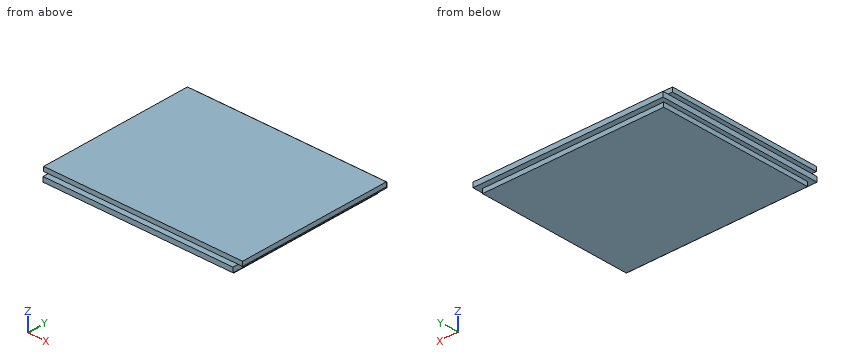
```python
from build123d import *

# Parameters (mm, degrees)
F0_W     = 114.3
F0_H     = 88.9
F1_DEPTH = 2.54
F2_W     = 109.22
F2_H     = 3.175
F2_H_2   = 88.9
F3_DEPTH = 2.794
F4_W     = 104.14
F4_H     = 88.9
F5_DEPTH = 2.54


with BuildPart() as f1:
    # F0 (on Top) → F1 (new body)
    with BuildSketch(Plane.XY):
        Rectangle(F0_W, F0_H)
    extrude(amount=-F1_DEPTH)

    # F2 (on face) → F3 (join)
    with BuildSketch(Plane(origin=(0, 0, -2.54), x_dir=(1, 0, 0), z_dir=(0, 0, -1))):
        with Locations((0, 46.0375)):
            Rectangle(F2_W, F2_H)
        Rectangle(F2_W, F2_H_2)
        with Locations((0, -46.0375)):
            Rectangle(F2_W, F2_H)
    extrude(amount=F3_DEPTH)

    # F4 (on face) → F5 (join)
    with BuildSketch(Plane(origin=(0, 0, -5.334), x_dir=(1, 0, 0), z_dir=(0, 0, -1))):
        Rectangle(F4_W, F4_H)
    extrude(amount=F5_DEPTH)


solid = f1.part
```
Model file for the job. Use its own axes, mm. Give positions to 0.01 mm unless a question says otherwise; leave off trailing zeros. Loops run counter-clockwise (first coordinate to the right, second up) from the corner with the lowest first, then second, coordinate; pieces in that order, holes last. Notation, with made-up numbers: (33.25, 88.5) -> (39.25, 88.5) arc R32 cw to (39.25, 116.5) -> close; hole circle Ø2 at (62.5, 3.5). An arc over 180 degrees is marked (long way). Write each question's results on one line, items separated by ' | '.
(1) Flat gauge pins, fed straight in: pin 1 Ø1.4 at (y, z) = (5.5, -4.5) entering from -X; pin 2 Ø0.8 at (y, z) = (1.5, -3.5) entering from +X; pin 3 Ø3 at (x, y) = (55.5, -0.5) entering from -Z. Where does each tip first touch, or does it go through?
Geometry results:
pin 1: stops at x = -54.61 | pin 2: stops at x = 54.61 | pin 3: stops at z = -5.33
(2) Cut at C-C on z = -1.25. List the corners of the cut face in (x, y), and give its area (3 significant figures).
Geometry results:
outline: (-57.15, -44.45) -> (57.15, -44.45) -> (57.15, 44.45) -> (-57.15, 44.45) -> close | area: 10,200 mm²
(3) Cut at B-B on x = -19. List the corners of the cut face in (y, z) (3 decimals), and give its area (3 significant figures).
Geometry results:
outline: (-47.625, -5.334) -> (-44.45, -5.334) -> (-44.45, -7.874) -> (44.45, -7.874) -> (44.45, -5.334) -> (47.625, -5.334) -> (47.625, -2.54) -> (44.45, -2.54) -> (44.45, 0) -> (-44.45, 0) -> (-44.45, -2.54) -> (-47.625, -2.54) -> close | area: 718 mm²
(4) Cut at A-A on y = -22. List the corners of the cut face in (x, z), and give its area (3 significant figures).
Geometry results:
outline: (-57.15, -2.54) -> (-54.61, -2.54) -> (-54.61, -5.33) -> (-52.07, -5.33) -> (-52.07, -7.87) -> (52.07, -7.87) -> (52.07, -5.33) -> (54.61, -5.33) -> (54.61, -2.54) -> (57.15, -2.54) -> (57.15, 0) -> (-57.15, 0) -> close | area: 860 mm²
(5) Probe line 1 along X through (y, z) = (1.5, -3.25); line 2 along Y through (x, z) = (-38, -1.25); line 3 along X through (y, z) = (33.5, -6.25). List the from-to ranges inside material, lowest first.
Geometry results:
line 1: x = -54.61 to 54.61 | line 2: y = -44.45 to 44.45 | line 3: x = -52.07 to 52.07
